Design review of the part shown in the three views and the two pictorial views. Dimensions are in mm from the part's minimum x, y and z. Round coordinates to 2 decimals unless told otherwise and drop trailing zeros. Order: outer loops, then holes, each group sorted by start corner. A loop starts at its lowest first (then second) coordinate and runs counter-clockwise, first axis right, second up.
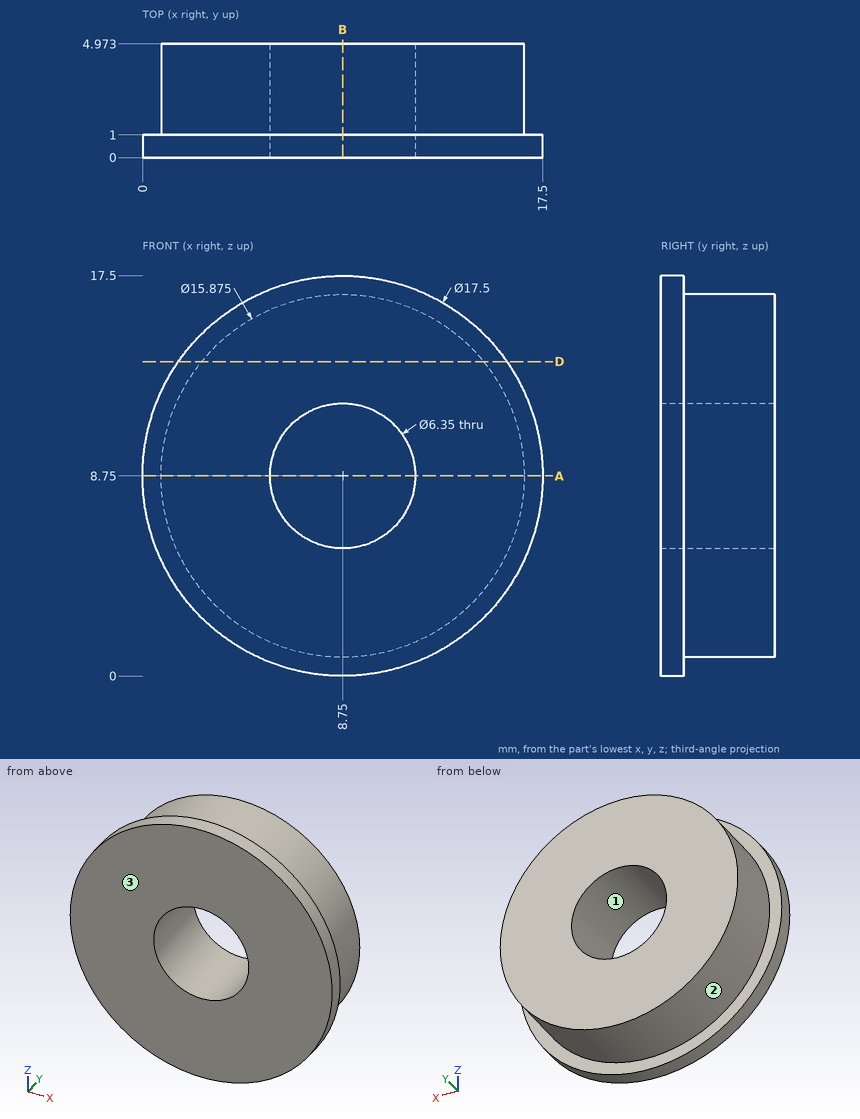
1) Take a section at D-D on z = 13.75. Give the boundary of the cut face in (x, y).
Results:
outline: (1.57, 0) - (15.93, 0) - (15.93, 1) - (14.91, 1) - (14.91, 4.97) - (2.59, 4.97) - (2.59, 1) - (1.57, 1) - close
2) Take a section at B-B on x = 8.75. Give the boundary of the cut face in (y, z) (1 decimal), plus the area to 3 significant figures.
Results:
outline: (0, 0) - (1, 0) - (1, 0.8) - (5, 0.8) - (5, 5.6) - (0, 5.6) - close; (0, 11.9) - (5, 11.9) - (5, 16.7) - (1, 16.7) - (1, 17.5) - (0, 17.5) - close
area: 49.0 mm2
3) To check wall thickness, follow line 1 along X through (y, z) = (3.8, 8.75) (1 decimal); line 2 along Z through (x, y) = (11.5, 4.6). State the ranges of each line that lie inside material, in increasing order.
Results:
line 1: x = 0.8 to 5.6, 11.9 to 16.7
line 2: z = 1.3 to 7.16, 10.34 to 16.2
4) Clearance check with flat-ended pins moving along their axes: P1, Ø1.5, axis at x = 11, y = 1, coming from the -Z side; P2, Ø2, axis at y = 1.5, z = 2.5, coming from the +X side; P3, Ø7.5, axis at x = 8.75, z = 8.75, coming from the +Y side; P4, Ø1.5, axis at y = 1.5, z = 7.5, coming from the +X side. State where each tip first meets the part, or that it passes through.
Results:
P1: stops at z = 0.13
P2: stops at x = 15.65
P3: stops at y = 4.97
P4: stops at x = 17.47
5) Take a section at A-A on z = 8.75. Give the boundary of the cut face in (x, y) (1 decimal), plus the area to 3 significant figures.
Results:
outline: (0, 0) - (5.6, 0) - (5.6, 5) - (0.8, 5) - (0.8, 1) - (0, 1) - close; (11.9, 0) - (17.5, 0) - (17.5, 1) - (16.7, 1) - (16.7, 5) - (11.9, 5) - close
area: 49.0 mm2
6) The part is to be moulded in two halves that separate along X. For the marked faces 1, 2 and 3, say which applies: released by +X, released by -X, zero draft, split by the parting line, or undercut.
Results:
face 1: undercut
face 2: split by the parting line
face 3: zero draft
